Input: part model. Units: mm. Frame: model coordinates. A direction names the side the tool comes from. Round coordinates to 2 decimals unless told otherwise and drop trailing zeros. Loops run counter-clockwise (first coordinate to the right, second up) from the corner with the lowest first, then second, coordinate; pieces in that order, holes last. Notation, with made-up numbers: M -28,41.25 L -9,41.25 A22 ccw -9,70.25 Z; hole C 77.5,-23 d11. An arc over 180 degrees is marked long. Put each result on its own line as item: value. Start each with the question number.
1) Draft query along X for faces 3 (the face through (6, 1, -12.065)), 4 (the face through (0, 1, -6)), 5 (the face through (12.7, 1, -6)), 6 (the face through (12.065, 1, -6)). Return one class per face: +X half, -X half, draft (parallel to the pull), parting line (faces both ways), or undercut.
2) Section B-B on z = -10. Output: boundary loops of the cut face in (x, y) (3 decimals), plus the area to 3 significant figures.
3) Pin query (flat end, axial travel): pin 1 (1 mm diameter, centred on x = 5, z = -11, fed in from -Y) (3 decimals). Return the tip coordinate at first contact, or that it passes through.
4) Line query: probe 1 along Z at (x, y) = (11, 1.85) (3 decimals); probe 2 along X at (y, z) = (1.85, -10.75) (3 decimals); probe 3 along X at (y, z) = (1.4, -5) (3 decimals). Output: solid intervals per line, ascending.
5) Section A-A on y = 1.3. Output: boundary loops of the cut face in (x, z) (3 decimals).
6) Reachability of faces 1 (the face through (7, 2.543, -6)), 2 (the face through (8.83, 0.97, -6.9)) from +Z, -Z, +X, -X, +Y, -Y: full face, straight path, thin tool, end or side. Return the list, or none.
7) Section C-C on x = 7.75. Output: boundary loops of the cut face in (y, z) (3 decimals).
from build123d import *

# Parameters (mm, degrees)
SKETCH1_W           = 12.7
SKETCH1_H           = 12.7
BOSS_EXTRUDE1_DEPTH = 2.54
FILLET1_R           = 0.635
SHELL1_START        = 0.635
SHELL1_OUTLINE_W    = 1.905
SHELL1_OUTLINE_H    = 11.43
SHELL1_DEPTH        = 11.43
SKETCH2_R           = 2.54
BOSS_EXTRUDE2_DEPTH = 1.905
BOSS_EXTRUDE3_DEPTH = 0.00254


# Read off the part's stored shape, not the designer's step: Shell1
with BuildPart() as part:
    # Sketch1 → Boss-Extrude1 (new body)
    with BuildSketch(Plane(origin=(0, 0, 0), x_dir=(1, 0, 0), z_dir=(0, 1, 0))):
        with Locations((6.35, 6.35)):
            Rectangle(SKETCH1_W, SKETCH1_H)
    extrude(amount=BOSS_EXTRUDE1_DEPTH)

    # Fillet1
    fillet1_edges = [part.edges().sort_by_distance(p)[0] for p in [
        (0, 1.27, -12.7),
        (12.7, 1.27, -12.7),
        (12.7, 1.27, 0),
        (0, 1.27, 0),
    ]]
    fillet(fillet1_edges, radius=FILLET1_R)

    # Shell1 outline → Shell1 (cut)
    with BuildSketch(Plane.YZ.offset(SHELL1_START)):
        with Locations((0.9525, -6.35)):
            Rectangle(SHELL1_OUTLINE_W, SHELL1_OUTLINE_H)
    extrude(amount=SHELL1_DEPTH, mode=Mode.SUBTRACT)

    # Sketch2 → Boss-Extrude2 (add)
    with BuildSketch(Plane(origin=(0, 1.905, 0), x_dir=(-1, 0, 0), z_dir=(0, -1, 0))):
        with Locations(Location((-6.35, 6.35, 0), (0, 0, 270))):
            Circle(SKETCH2_R)
    extrude(amount=BOSS_EXTRUDE2_DEPTH)

    # Sketch3 → Boss-Extrude3 (add)
    with BuildSketch(Plane(origin=(0, 2.54, 0), x_dir=(1, 0, 0), z_dir=(0, 1, 0))):
        with BuildLine():
            Line((5.192346154, 8.001), (5.762217949, 8.001))
            Line((5.762217949, 8.001), (5.762217949, 5.935214744))
            add(Edge.make_bspline(
                [(5.762217949, 5.935214744), (5.762248936, 5.913797578), (5.762308786, 5.872430544), (5.765304944, 5.813082394), (5.768046636, 5.758529018), (5.772993425, 5.70883014), (5.780301528, 5.663964501), (5.787378157, 5.6236439), (5.796955674, 5.588590232), (5.811349151, 5.54868998), (5.833524775, 5.503859868), (5.869758513, 5.457136896), (5.911569146, 5.414495403), (5.961681599, 5.37900224), (6.018003565, 5.35029147), (6.080225578, 5.329019967), (6.148259929, 5.317195835), (6.195301951, 5.315390665), (6.219514623, 5.314461538)],
                knots=[0, 0, 0, 0, 1.155499968, 2.231836252, 3.205919964, 4.102923608, 4.924856345, 5.658536265, 6.31071849, 6.882491295, 7.94666036, 8.992281882, 10.060072772, 11.158554251, 12.289267114, 13.461410017, 14.693379945, 16, 16, 16, 16], degree=3))
            add(Edge.make_bspline(
                [(6.219514623, 5.314461538), (6.2452376, 5.315212154), (6.29539305, 5.316675726), (6.367533681, 5.331042272), (6.434372384, 5.353918735), (6.494493956, 5.386569277), (6.547838568, 5.425706674), (6.592993664, 5.47033557), (6.628629899, 5.520544979), (6.651856272, 5.566866983), (6.664896736, 5.609502353), (6.674671214, 5.647595439), (6.681836988, 5.692541509), (6.688338013, 5.743638634), (6.692244628, 5.801416082), (6.696480716, 5.865409199), (6.698033281, 5.936055843), (6.698297904, 5.985248427), (6.698435897, 6.010900841)],
                knots=[0, 0, 0, 0, 1.261321664, 2.459363699, 3.594844139, 4.716940403, 5.803436589, 6.833651888, 7.818396249, 8.814403945, 9.360733334, 10.004355033, 10.743453831, 11.592799886, 12.532235708, 13.585170094, 14.740740724, 16, 16, 16, 16], degree=3))
            Line((6.698435897, 6.010900841), (6.698435897, 8.001))
            Line((6.698435897, 8.001), (7.268307692, 8.001))
            Line((7.268307692, 8.001), (7.268307692, 6.106939503))
            add(Edge.make_bspline(
                [(7.268307692, 6.106939503), (7.268228555, 6.068565928), (7.268076382, 5.994777286), (7.265739466, 5.888737813), (7.260764595, 5.791887765), (7.256586276, 5.704198842), (7.2484998, 5.625789174), (7.240075588, 5.55632393), (7.229338205, 5.49604928), (7.213361625, 5.427433916), (7.185790778, 5.348425837), (7.141342957, 5.257451459), (7.084919326, 5.168382033), (7.018229414, 5.082197383), (6.942930403, 5.00213462), (6.860691833, 4.931849878), (6.772820271, 4.872396565), (6.678397522, 4.825228387), (6.577503944, 4.788440763), (6.469141271, 4.763721333), (6.353383397, 4.747020576), (6.273427246, 4.745416263), (6.232234976, 4.744589744)],
                knots=[0, 0, 0, 0, 1.170808336, 2.251350247, 3.235597562, 4.129743112, 4.929140599, 5.639994148, 6.264258765, 6.79612947, 7.788252245, 8.809469599, 9.879094798, 10.999557536, 12.129761673, 13.226370002, 14.293821979, 15.358369427, 16.438775801, 17.562147481, 18.744053101, 20, 20, 20, 20], degree=3))
            add(Edge.make_bspline(
                [(6.232234976, 4.744589744), (6.204866012, 4.745050738), (6.150867608, 4.745960269), (6.071453481, 4.753979964), (5.994684128, 4.765797979), (5.920703797, 4.783039245), (5.849255717, 4.80531174), (5.780358869, 4.832727631), (5.714269291, 4.865133995), (5.65135681, 4.902232764), (5.591698847, 4.942348696), (5.537174548, 4.986818895), (5.485907605, 5.032354622), (5.439379097, 5.080872214), (5.397239555, 5.131862319), (5.359575764, 5.185440497), (5.326443681, 5.24160199), (5.297009886, 5.301359104), (5.27181743, 5.367749078), (5.250579243, 5.443133431), (5.232025064, 5.528693737), (5.218236692, 5.624622759), (5.205736074, 5.730604326), (5.197823871, 5.846914536), (5.193684642, 5.973556726), (5.19280359, 6.061355131), (5.192346154, 6.106939503)],
                knots=[0, 0, 0, 0, 1.001158378, 1.975264943, 2.917723546, 3.841610987, 4.75185031, 5.653588123, 6.552117133, 7.442167995, 8.324307438, 9.179605724, 10.014504199, 10.831958861, 11.636465792, 12.43274043, 13.225645099, 14.020104002, 14.867201867, 15.819789774, 16.883317127, 18.068162734, 19.364263498, 20.787406516, 22.332041935, 24, 24, 24, 24], degree=3))
            Line((5.192346154, 6.106939503), (5.192346154, 8.001))
        make_face()
    extrude(amount=BOSS_EXTRUDE3_DEPTH)


solid = part.part
Geometry results:
1. face 3: undercut
1. face 4: -X half
1. face 5: +X half
1. face 6: undercut
2. outline: M 0,0 L 0.635,0 L 0.635,1.905 L 12.065,1.905 L 12.065,0 L 12.7,0 L 12.7,2.54 L 0,2.54 Z
2. area: 10.5 mm²
3. pin 1: stops at y = 1.905
4. probe 1: z = -12.7 to -12.065, -0.635 to 0
4. probe 2: x = 0 to 0.635, 12.065 to 12.7
4. probe 3: x = 0 to 0.635, 4.198 to 8.502, 12.065 to 12.7
5. outline: M 0,-12.065 A0.635 ccw 0.635,-12.7 L 12.065,-12.7 A0.635 ccw 12.7,-12.065 L 12.7,-0.635 A0.635 ccw 12.065,0 L 0.635,0 A0.635 ccw 0,-0.635 Z; C 6.35,-6.35 d5.08; hole M 0.635,-12.065 L 12.065,-12.065 L 12.065,-0.635 L 0.635,-0.635 Z
6. face 1: +Z, -Z, +X, -X, +Y
6. face 2: -Y
7. outline: M 0,-12.7 L 2.54,-12.7 L 2.54,0 L 0,0 L 0,-0.635 L 1.905,-0.635 L 1.905,-4.231 L 0,-4.231 L 0,-8.469 L 1.905,-8.469 L 1.905,-12.065 L 0,-12.065 Z
